Autodesk Inventor part; units mm, degrees
ref_plane "YZ Plane" through (0, 0, 0) normal (1, 0, 0) x (0, 1, 0)
ref_plane "XZ Plane" through (0, 0, 0) normal (0, 1, 0) x (-1, 0, 0)
ref_plane "XY Plane" through (0, 0, 0) normal (0, 0, 1) x (1, 0, 0)
sketch "Sketch1" plane through (0, 0, 0) normal (0, 0, 1) x (1, 0, 0)
  line L0 (-32.5, 32.5) -> (32.5, 32.5) construction
  line L1 (32.5, 32.5) -> (32.5, -32.5) construction
  line L2 (32.5, -32.5) -> (-32.5, -32.5) construction
  line L3 (-32.5, -32.5) -> (-32.5, 32.5) construction
  circle A0 centre (-32.5, 32.5) radius 2.5
  circle A1 centre (32.5, 32.5) radius 2.5
  circle A2 centre (-32.5, -32.5) radius 2.5
  circle A3 centre (32.5, -32.5) radius 2.5
  line L4 (-32.5, 32.5) -> (32.5, -32.5) construction
  circle A4 centre (0, 0) radius 10
  circle A5 centre (-32.5, 32.5) radius 4.25
  circle A6 centre (32.5, 32.5) radius 4.25
  circle A7 centre (-32.5, -32.5) radius 4.25
  circle A8 centre (32.5, -32.5) radius 4.25
  line L5 (-32.5, 36.75) -> (32.5, 36.75)
  line L6 (32.5, -36.75) -> (-32.5, -36.75)
  line L7 (-36.75, 32.5) -> (-36.75, -32.5)
  line L8 (36.75, 32.5) -> (36.75, -32.5)
  dimension "d1" = 65
  dimension "d2" = 5
  dimension "d4" = 20
  dimension "d16" = 8.5
extrude "Extrusion1" add sketch "Sketch1" along normal blind 4
sketch "Sketch2" plane through (0, 0, 4) normal (0, 0, 1) x (1, 0, 0)
  line L0 (-11.2, 11.2) -> (11.2, 11.2)
  line L1 (11.2, -11.2) -> (-11.2, -11.2)
  line L2 (0, 11.2) -> (0, 36.75) construction
  line L3 (0, -11.2) -> (0, -36.75) construction
  line L4 (-13.2, 13.2) -> (13.2, 13.2)
  line L5 (13.2, -13.2) -> (-13.2, -13.2)
  line L6 (11.2, 11.2) -> (13.2, 13.2) construction
  line L7 (-11.2, 11.2) -> (-13.2, 13.2) construction
  line L8 (-13.2, -13.2) -> (-11.2, -11.2) construction
  line L9 (11.2, -11.2) -> (13.2, -13.2) construction
  circle A0 centre (0, 0) radius 10
  circle A1 centre (-32.5, -32.5) radius 2.5
  circle A2 centre (32.5, -32.5) radius 2.5
  circle A3 centre (32.5, 32.5) radius 2.5
  circle A4 centre (-32.5, 32.5) radius 2.5
  arc A5 (32.5, -36.75) -> (36.75, -32.5) centre (32.5, -32.5) ccw
  line L10 (36.75, -32.5) -> (36.75, 32.5)
  arc A6 (36.75, 32.5) -> (32.5, 36.75) centre (32.5, 32.5) ccw
  line L11 (32.5, 36.75) -> (-32.5, 36.75)
  arc A7 (-32.5, 36.75) -> (-36.75, 32.5) centre (-32.5, 32.5) ccw
  line L12 (-36.75, 32.5) -> (-36.75, -32.5)
  arc A8 (-36.75, -32.5) -> (-32.5, -36.75) centre (-32.5, -32.5) ccw
  line L13 (-32.5, -36.75) -> (32.5, -36.75)
  line L14 (-32.5, -36.75) -> (32.5, -36.75)
  line L15 (36.75, -32.5) -> (36.75, 32.5)
  line L16 (32.5, 36.75) -> (-32.5, 36.75)
  line L17 (-13.2, 10) -> (-11.2, 10)
  line L18 (-13.2, -10) -> (-11.2, -10)
  line L19 (-13.2, -13.2) -> (-13.2, -10)
  line L20 (-13.2, 10) -> (-13.2, 13.2)
  line L21 (-11.2, -11.2) -> (-11.2, -10)
  line L22 (-11.2, 10) -> (-11.2, 11.2)
  line L23 (11.2, 10) -> (13.2, 10)
  line L24 (11.2, -10) -> (13.2, -10)
  line L25 (11.2, 11.2) -> (11.2, 10)
  line L26 (11.2, -10) -> (11.2, -11.2)
  line L27 (13.2, 13.2) -> (13.2, 10)
  line L28 (13.2, -10) -> (13.2, -13.2)
  line L29 (-11.2, 11.2) -> (0, 0) construction
  line L30 (0, 0) -> (-11.2, -11.2) construction
  line L31 (0, 0) -> (11.2, 11.2) construction
  line L32 (0, 0) -> (11.2, -11.2) construction
  dimension "d7" = 22.4
  dimension "d24" = 2
  dimension "d31" = 2
  dimension "d34" = 20
extrude "Extrusion2" add sketch "Sketch2" along normal blind 2 contours L22 L17 L20 L4 L27 L23 L25 L0 | L26 L24 L28 L5 L19 L18 L21 L1
extrude "Extrusion4" add sketch "Sketch1" along normal blind 6 contours A5 | A6 | A7 | A8
sketch "Sketch4" plane through (0, 0, 4) normal (0, 0, 1) x (1, 0, 0)
  line L0 (13.2, 13.2) -> (13.2, 10)
  line L1 (-13.2, 13.2) -> (13.2, 13.2)
  arc A0 (36.75, -32.5) -> (32.5, -36.75) centre (32.5, -32.5) ccw
  line L2 (36.75, -32.5) -> (36.75, 32.5)
  arc A1 (32.5, 36.75) -> (36.75, 32.5) centre (32.5, 32.5) ccw
  line L3 (32.5, 36.75) -> (-32.5, 36.75)
  arc A2 (-36.75, 32.5) -> (-32.5, 36.75) centre (-32.5, 32.5) ccw
  line L4 (-36.75, 32.5) -> (-36.75, -32.5)
  arc A3 (-32.5, -36.75) -> (-36.75, -32.5) centre (-32.5, -32.5) ccw
  line L5 (-32.5, -36.75) -> (32.5, -36.75)
  line L6 (-13.2, 10) -> (-13.2, -10)
  line L7 (-13.2, -10) -> (-36.75, -10)
  line L8 (-36.75, -10) -> (-36.75, 10)
  line L9 (-36.75, 10) -> (-13.2, 10)
  line L10 (32.5, 36.75) -> (-32.5, 36.75) construction
  line L11 (0, 36.75) -> (0, -36.75) construction
  line L12 (13.2, 10) -> (13.2, -10)
  line L13 (13.2, -10) -> (36.75, -10)
  line L14 (36.75, -10) -> (36.75, 10)
  line L15 (36.75, 10) -> (13.2, 10)
  line L16 (-11.2, 11.2) -> (-11.2, 10)
  line L17 (-11.2, 10) -> (-13.2, 10)
  line L18 (-13.2, 10) -> (-13.2, 13.2)
  line L19 (13.2, 10) -> (11.2, 10)
  line L20 (11.2, 10) -> (11.2, 11.2)
  line L21 (11.2, 11.2) -> (-11.2, 11.2)
  line L22 (-11.2, 11.2) -> (11.2, 11.2)
  line L23 (11.2, 11.2) -> (11.2, 10)
  line L24 (11.2, 10) -> (13.2, 10)
  line L25 (13.2, 10) -> (13.2, 13.2)
  line L26 (13.2, 13.2) -> (-13.2, 13.2)
  line L27 (-13.2, 13.2) -> (-13.2, 10)
  line L28 (-13.2, 10) -> (-11.2, 10)
  line L29 (-11.2, 10) -> (-11.2, 11.2)
  line L30 (-11.2, -11.2) -> (-11.2, -10)
  line L31 (-13.2, -10) -> (-13.2, -13.2)
  line L32 (-13.2, 13.2) -> (-13.2, 10)
  circle A4 centre (0, 0) radius 10
  line L33 (-11.2, -11.2) -> (11.2, -11.2)
  line L34 (11.2, -11.2) -> (11.2, -10)
  line L35 (11.2, -10) -> (13.2, -10)
  line L36 (13.2, -10) -> (13.2, -13.2)
  line L37 (13.2, -13.2) -> (-13.2, -13.2)
  line L38 (-13.2, -13.2) -> (-13.2, -10)
  line L39 (-13.2, -10) -> (-11.2, -10)
  line L40 (-11.2, -10) -> (-11.2, -11.2)
  point P0 (-36.75, 0)
  point P1 (36.75, 0)
  dimension "d20" = 20
extrude "Extrusion5" cut sketch "Sketch4" against normal through all contours L15 L2 L13 L12 | L6 L7 L4 L9
properties part number "20mm glass cuvette holder"
Could you check a few things on this model? Use its own coordinates, in mm. A direction names the side the tool comes from. Round coordinates to 2 decimals unless told otherwise and drop trailing zeros. Write each loop counter-clockwise with the first axis right and the second up, starting at its lowest first coordinate (ties: lowest second). Pieces come first, ordered by that corner, then holes. Notation, with made-up numbers: (-4, 5.5) -> (18, 5.5) arc R23 cw to (18, 26.5) -> close; hole circle Ø2 at (52.25, -19). An arc over 180 degrees is marked (long way). Use a Markdown table: item, result.
1. If we section it at C-C (y = 0): List the corners of the cut face in (x, z) for me, then the cut area to 3 significant figures.
Answer key:
| item | result |
|---|---|
| outline | (-13.2, 0) -> (-10, 0) -> (-10, 4) -> (-13.2, 4) -> close; (10, 0) -> (13.2, 0) -> (13.2, 4) -> (10, 4) -> close |
| area | 25.6 mm^2 |
2. If we section it at D-D (x = 22.5): List the corners of the cut face in (y, z) for me.
Answer key:
| item | result |
|---|---|
| outline | (-36.75, 0) -> (-10, 0) -> (-10, 4) -> (-36.75, 4) -> close; (10, 0) -> (36.75, 0) -> (36.75, 4) -> (10, 4) -> close |
3. Which directions (+Z, -Z, +X, -X, +Y, -Y) give clear straight access to the entire face, cutting with the end or side of a thin tool? Please do faces 1 (the face through (0, -11.2, 5)), 2 (the face through (-13.2, 0, 2)), 3 (the face through (0, 13.2, 5)), 4 (the face through (-12, -10, 5)), 5 (the face through (13.2, 12, 5)).
Answer key:
| item | result |
|---|---|
| face 1 | +Z |
| face 2 | +Z, -Z, -X |
| face 3 | +Z, +X, -X, +Y |
| face 4 | +Z, +X, -X |
| face 5 | +Z, +X, +Y, -Y |
4. If we section it at A-A (z = 5): State how many separate pieces and enclosed holes the cut face has, then the cut area to 3 significant figures.
Answer key:
| item | result |
|---|---|
| separate pieces | 6 |
| enclosed holes | 4 |
| area | 264 mm^2 |
5. For pin 1 Ø1.2 at (y, z) = (0.5, 2) entering from -X; pin 2 Ø1.5 at (x, y) = (4.5, 26.5) entering from +Z; pin 3 Ø1 at (x, z) = (12.5, 5.5) entering from -Y, each with a flat end and sliding along its axis, tell me the tip position at first contact or that it passes through.
Answer key:
| item | result |
|---|---|
| pin 1 | stops at x = -13.2 |
| pin 2 | stops at z = 4 |
| pin 3 | stops at y = -13.2 |
6. If we section it at B-B (x = 0): List the corners of the cut face in (y, z) for me, then the cut area to 3 significant figures.
Answer key:
| item | result |
|---|---|
| outline | (-36.75, 0) -> (-10, 0) -> (-10, 4) -> (-11.2, 4) -> (-11.2, 6) -> (-13.2, 6) -> (-13.2, 4) -> (-36.75, 4) -> close; (10, 0) -> (36.75, 0) -> (36.75, 4) -> (13.2, 4) -> (13.2, 6) -> (11.2, 6) -> (11.2, 4) -> (10, 4) -> close |
| area | 222 mm^2 |
7. Please list where these lines run through material, in increasing order: probe 1 along Y at (x, z) = (-32.5, 2.7); probe 2 along Y at (x, z) = (-12.5, 5.1).
Answer key:
| item | result |
|---|---|
| probe 1 | y = -36.75 to -35, -30 to -10, 10 to 30, 35 to 36.75 |
| probe 2 | y = -13.2 to -10, 10 to 13.2 |
